For this review, take the finished solid that the model builds, in its own axes (mm). Face numbers are marked on the shaded views. A direction names the side the tool comes from. Give positions to 0.01 mm unless a question says otherwise; leave off trailing zeros. Write each loop counter-clockwise with the first axis right and the second up, starting at its lowest first coordinate (ties: lowest second). Pieces come first, ordered by that corner, then holes.
Q1. Mouldability with a two-part tool opening along Y and no side actions: class the marked faces 4, 5 and 6 as released by +Y, released by -Y, zero draft, split by the parting line, or undercut.
Q2. We need section D-D (z = 2.75). Write out the cut boundary in (x, y), then the cut area to 3 significant figures.
Q3. Insertion check: P1, Ø1.5, axis at y = 12, z = -2.5, coming from the -X side; P2, Ø4, axis at x = -2, z = 2, coming from the +Y side; P3, Ø1, axis at x = -0.5, y = 4, coming from the -Z side; P4, Ø3, axis at x = 2.5, y = 12.5, coming from the +Z side. Each pin has a flat end and moves straight along its axis. Give the tip position at first contact, or say it passes through.
Q4. We need section C-C (y = 8.75). Write out the cut boundary in (x, z).
Q5. For line 1 (Z direction, x = 0, y = 11.5); line 2 (Z direction, x = 0, y = 5.5); line 3 (X direction, y = 6, z = 0.5), list the stretches that pass through material, from the lowest coordinate up.
Q6. Machinability: for the marked faces 1, 2 and 3, which of the approach directions +Z, -Z, +X, -X, +Y, -Y give a long, thin tool a straight path to every point of the face, cutting with its end or side? Answer none if there is none.
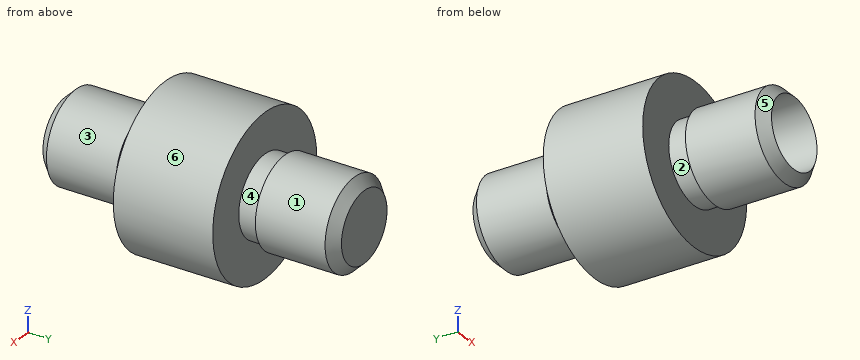
Autodesk Inventor part; units mm, degrees
ref_plane "Work Plane4" through (0, 7.5, 0) normal (0, 1, 0) x (-1, 0, 0)
ref_plane "YZ Plane" through (0, 0, 0) normal (1, 0, 0) x (0, 1, 0)
ref_plane "XY Plane" through (0, 0, 0) normal (0, 0, 1) x (1, 0, 0)
sketch "Sketch1" plane through (0, 0, 0) normal (0, 1, 0) x (-1, 0, 0)
  circle A0 centre (0, 0) radius 1.75
  circle A1 centre (0, 0) radius 2
  dimension "d0" = 3.5
  dimension "d1" = 4
extrude "Extrusion1" add sketch "Sketch1" along normal blind 15
sketch "Sketch2" plane through (0, 0, 0) normal (0, -1, 0) x (1, 0, 0)
  circle A0 centre (0, 0) radius 2.25
  circle A1 centre (0, 0) radius 2
  dimension "d4" = 4.5
extrude "Extrusion2" add sketch "Sketch2" against normal blind 4
sketch "Sketch3" plane through (0, 15, 0) normal (0, 1, 0) x (1, 0, 0)
  circle A0 centre (0, 0) radius 2
  circle A1 centre (0, 0) radius 2.25
  circle A2 centre (0, 0) radius 2.25
  dimension "d9" = 4.5
  dimension "d10" = 4.5
  dimension "d11" = 4
  dimension "d12" = 0
extrude "Extrusion3" add sketch "Sketch3" against normal blind 4
ref_plane "Work Plane4" through (0, 7.5, 0) normal (0, 1, 0) x (-1, 0, 0)
ref_plane "Work Plane3" through (0, -4, 0) normal (0, 1, 0) x (-1, 0, 0)
sketch "Sketch4" plane through (0, 7.5, 0) normal (0, 1, 0) x (-1, 0, 0)
  circle A0 centre (0, 0) radius 2
  circle A1 centre (0, 0) radius 4
  dimension "d16" = 4
  dimension "d17" = 8
chamfer "Chamfer3" distance 0.5 angle 45 1 edges at (-2.25, 0, 0)
chamfer "Chamfer4" distance 0.5 angle 45 1 edges at (-2.25, 15, 0)
extrude "Extrusion5" add sketch "Sketch4" along normal mid plane 5
properties part number "reverse gear cylinder piping connector 2"
Computed:
1. face 4: undercut
1. face 5: released by -Y
1. face 6: zero draft
2. outline: (-2.9, 5) - (2.9, 5) - (2.9, 10) - (-2.9, 10) - close
2. area: 29.0 mm2
3. P1: stops at x = -1.41
3. P2: stops at y = 15
3. P3: stops at z = -2.25
3. P4: stops at z = 2.02
4. outline: circle Ø8 at (0, 0); hole circle Ø3.5 at (0, 0)
5. line 1: z = -2.25 to -1.75, 1.75 to 2.25
5. line 2: z = -4 to -1.75, 1.75 to 4
5. line 3: x = -3.97 to -1.68, 1.68 to 3.97
6. face 1: +Y
6. face 2: none
6. face 3: -Y
